```python
from build123d import *

# Parameters (mm, degrees)
SKETCH1_W           = 600
SKETCH1_H           = 300
BOSS_EXTRUDE1_DEPTH = 30
CUT_EXTRUDE1_DEPTH  = 672.490878568
FILLET1_R           = 25
FILLET2_R           = 10
SKETCH3_W           = 195
SKETCH3_H           = 250
CUT_EXTRUDE2_DEPTH  = 672.490878568
SKETCH4_R           = 3.25
CUT_EXTRUDE3_DEPTH  = 200
CUT_EXTRUDE4_DEPTH  = 3
SKETCH7_R           = 4.66700581
CUT_EXTRUDE5_DEPTH  = 53
SKETCH8_R           = 3.25
CUT_EXTRUDE6_DEPTH  = 53
FILLET3_R           = 13
FILLET4_R           = 5


with BuildPart() as part:
    # Sketch1 → Boss-Extrude1 (new body)
    with BuildSketch(Plane(origin=(0, 0, 0), x_dir=(1, 0, 0), z_dir=(0, 1, 0))):
        with Locations((300, 150)):
            Rectangle(SKETCH1_W, SKETCH1_H)
    extrude(amount=BOSS_EXTRUDE1_DEPTH)

    # Sketch2 → Cut-Extrude1 (cut, through all)
    with BuildSketch(Plane(origin=(0, 30, 0), x_dir=(1, 0, 0), z_dir=(0, 1, 0))):
        with BuildLine():
            Line((225, 350), (375, 350))
            Line((375, 350), (375, 260))
            ThreePointArc((375, 260), (372.071067812, 252.928932188), (365, 250))
            Line((365, 250), (235, 250))
            ThreePointArc((235, 250), (227.928932188, 252.928932188), (225, 260))
            Line((225, 260), (225, 350))
        make_face()
    extrude(amount=-CUT_EXTRUDE1_DEPTH, mode=Mode.SUBTRACT)

    # Fillet1
    fillet1_edges = [part.edges().sort_by_distance(p)[0] for p in [
        (300, 30, 0),
    ]]
    fillet(fillet1_edges, radius=FILLET1_R)

    # Fillet2
    fillet2_edges = [part.edges().sort_by_distance(p)[0] for p in [
        (487.5, 30, -300),
        (112.5, 30, -300),
        (600, 30, -162.5),
        (600, 2.5, 0),
        (600, 22.67766953, -7.32233047),
        (0, 2.5, 0),
        (0, 22.67766953, -7.32233047),
        (0, 30, -162.5),
    ]]
    fillet(fillet2_edges, radius=FILLET2_R)

    # Sketch3 → Cut-Extrude2 (cut, through all)
    with BuildSketch(Plane(origin=(0, 30, 0), x_dir=(1, 0, 0), z_dir=(0, 1, 0))):
        Polygon((280, 240), (280, 220), (320, 220), (320, 240), (375, 240), (375, 30), (320, 30), (320, 50), (280, 50), (280, 30), (225, 30), (225, 240), align=None)
        with Locations((112.5, 155)):
            Rectangle(SKETCH3_W, SKETCH3_H)
        with Locations((487.5, 155)):
            Rectangle(SKETCH3_W, SKETCH3_H)
    extrude(amount=-CUT_EXTRUDE2_DEPTH, mode=Mode.SUBTRACT)

    # Sketch4 → Cut-Extrude3 (cut)
    with BuildSketch(Plane.ZY.offset(-210)):
        with Locations((-135.475660035, 15)):
            Circle(SKETCH4_R)
        with Locations((-85.475660035, 15)):
            Circle(SKETCH4_R)
    extrude(amount=-CUT_EXTRUDE3_DEPTH, mode=Mode.SUBTRACT)

    # Sketch6 → Cut-Extrude4 (cut)
    with BuildSketch(Plane(origin=(0, 30, 0), x_dir=(1, 0, 0), z_dir=(0, 1, 0))):
        with BuildLine():
            Line((10, 25), (590, 25))
            Line((590, 25), (590, 290))
            Line((590, 290), (375, 290))
            Line((375, 290), (375, 260))
            ThreePointArc((375, 260), (372.071067812, 252.928932188), (365, 250))
            Line((365, 250), (235, 250))
            ThreePointArc((235, 250), (227.928932188, 252.928932188), (225, 260))
            Line((225, 260), (225, 290))
            Line((225, 290), (10, 290))
            Line((10, 290), (10, 25))
        make_face()
    extrude(amount=-CUT_EXTRUDE4_DEPTH, mode=Mode.SUBTRACT)

    # Sketch7 → Cut-Extrude5 (cut)
    with BuildSketch(Plane.ZY.offset(-280)):
        with Locations((-230, 13.5)):
            Circle(SKETCH7_R)
        with Locations((-40, 13.5)):
            Circle(SKETCH7_R)
    extrude(amount=-CUT_EXTRUDE5_DEPTH, mode=Mode.SUBTRACT)

    # Sketch8 → Cut-Extrude6 (cut)
    with BuildSketch(Plane(origin=(0, 0, -250), x_dir=(-1, 0, 0), z_dir=(0, 0, -1))):
        with Locations((-335, 18)):
            Circle(SKETCH8_R)
        with Locations((-265, 18)):
            Circle(SKETCH8_R)
    extrude(amount=-CUT_EXTRUDE6_DEPTH, mode=Mode.SUBTRACT)

    # Fillet3
    fillet3_edges = [part.edges().sort_by_distance(p)[0] for p in [
        (390, 13.5, -30),
        (390, 13.5, -280),
        (585, 13.5, -280),
        (585, 13.5, -30),
        (15, 13.5, -30),
        (15, 13.5, -280),
        (210, 13.5, -280),
        (210, 13.5, -30),
        (225, 13.5, -240),
        (375, 13.5, -240),
        (375, 13.5, -30),
        (225, 13.5, -30),
    ]]
    fillet(fillet3_edges, radius=FILLET3_R)

    # Fillet4
    fillet4_edges = [part.edges().sort_by_distance(p)[0] for p in [
        (280, 27, -230),
        (300, 27, -220),
        (320, 27, -230),
        (341, 27, -240),
        (320, 27, -40),
        (300, 27, -50),
        (280, 27, -40),
        (259, 27, -30),
        (375, 27, -135),
        (390, 27, -155),
        (487.5, 27, -280),
        (585, 27, -155),
        (487.5, 27, -30),
        (341, 27, -30),
        (225, 27, -135),
        (259, 27, -240),
        (210, 27, -155),
        (112.5, 27, -30),
        (15, 27, -155),
        (112.5, 27, -280),
        (371.192388155, 27, -236.192388155),
        (393.807611845, 27, -276.192388155),
        (581.192388155, 27, -276.192388155),
        (581.192388155, 27, -33.807611845),
        (393.807611845, 27, -33.807611845),
        (371.192388155, 27, -33.807611845),
        (228.807611845, 27, -236.192388155),
        (228.807611845, 27, -33.807611845),
        (206.192388155, 27, -33.807611845),
        (18.807611845, 27, -33.807611845),
        (18.807611845, 27, -276.192388155),
        (206.192388155, 27, -276.192388155),
    ]]
    fillet(fillet4_edges, radius=FILLET4_R - 0.0001)  # a hair under: the kernel refuses the full size


solid = part.part
```
For this review, take the finished solid that the model builds, in its own axes (mm). A direction names the side the tool comes from. Give positions to 0.01 mm unless a question says otherwise; leave off trailing zeros.
1) The part is to be moulded in two halves that separate along Z. For faces 4 (the face through (300, 11, -220)), 5 (the face through (387, 0, -140)), 6 (the face through (301, 14, -250)), say which applies: released by +Z, released by -Z, zero draft, split by the parting line, or undercut.
2) Insertion check: pin 1 (6 mm diameter, centred on x = 335, y = 18, fed in from +Z); pin 2 (4 mm diameter, centred on x = 265, y = 18, fed in from +Z); pin 3 (3.5 mm diameter, centred on x = 258.5, y = 29, fed in from -Z). Each pin has a flat end and moves straight along its axis. Give the tip position at first contact, or say it passes through.
3) Take a section at A-A (z = -175). State how many separate pieces and enclosed holes the cut face has, then the cut area to 3 significant figures.
4) Wall thickness on line 1 (X direction, y = 5, z = -145); line 2 (X direction, y = 15, z = -85); line 3 (X direction, y = 24.5, z = -276.5): over which ranges is each line inside the solid? List them lowest first.
5) For faces 1 (the face through (0, 10, -153)), 2 (the face through (342, 27, -246)), 3 (the face through (259, 11, -30)), list the 3-axis set-ups (+Z, -Z, +X, -X, +Y, -Y) from which the entire face can be reached by the end or side of a thin tool; tool diameter is ignored.
Derived:
1. face 4: undercut
1. face 5: zero draft
1. face 6: released by -Z
2. pin 1: stops at z = -2.09
2. pin 2: stops at z = -2.55
2. pin 3: stops at z = -25
3. separate pieces: 4
3. enclosed holes: 0
3. area: 1,600 mm2
4. line 1: x = 0 to 15, 210 to 225, 375 to 390, 585 to 600
4. line 2: x = 0 to 15, 585 to 600
4. line 3: x = 1.07 to 18.17, 206.83 to 225, 375 to 393.17, 581.83 to 598.93
5. face 1: +Z, -Z, -X, +Y, -Y
5. face 2: +Y
5. face 3: +Y, -Y
